```python
from build123d import *

# Parameters (mm, degrees)
F0_W     = 46
F0_H     = 18
F0_W_2   = 40
F0_H_2   = 12
F1_DEPTH = 11
F2_W     = 40
F2_H     = 12
F3_DEPTH = 3
F4_R     = 1


with BuildPart() as f1:
    # F0 (on Top) → F1 (new body)
    with BuildSketch(Plane.XY):
        with Locations((23, 9)):
            Rectangle(F0_W, F0_H)
        with Locations((23, 9)):
            Rectangle(F0_W_2, F0_H_2, mode=Mode.SUBTRACT)
    extrude(amount=F1_DEPTH)

    # F2 (on Top) → F3 (join)
    with BuildSketch(Plane.XY):
        with Locations((23, 9)):
            Rectangle(F2_W, F2_H)
    extrude(amount=F3_DEPTH)

    # F4
    f4_edges = [f1.edges().sort_by_distance(p)[0] for p in [
        (46, 18, 5.5),
        (46, 0, 5.5),
        (0, 0, 5.5),
        (0, 18, 5.5),
        (23, 18, 11),
        (0, 9, 11),
        (23, 0, 11),
        (46, 9, 11),
    ]]
    fillet(f4_edges, radius=F4_R)


solid = f1.part
```
Source: CAD feature listing. Evaluate the final solid. Frame: model axes, mm. A direction names the side the tool comes from. Coordinates: 2 decimals unless noted, no trailing zeros. Loops run counter-clockwise (first coordinate to the right, second up) from the corner with the lowest first, then second, coordinate; pieces in that order, holes last. Notation, with made-up numbers: (21.5, 68) -> (64.5, 68) arc R23 cw to (64.5, 83) -> close; hole circle Ø5 at (-15, 58). An arc over 180 degrees is marked (long way). One line per item, written item: value. Start each with the question number.
Q1. Section query B-B, the plane x = 42.5. Return the cut outline in (y, z), and give its area (3 significant figures).
Q2. Set-up query: faces 4 (the face through (23, 18, 5)), 5 (the face through (23, 9, 3)). Return all of +Z, -Z, +X, -X, +Y, -Y with unobstructed straight access to the full face (end or side cutting, diameter ignored); none if empty.
Q3. Line query: line 1 along Y through (x, z) = (24, 10); line 2 along X through (y, z) = (4.5, 4.5); line 3 along Z through (x, y) = (24.5, 13.5). Output: solid intervals per line, ascending.
Q4. Section query C-C, the plane y = 5.25. Return the cut outline in (x, z).
Q5. Contact query for flat-ended pins moving along their axis: P1, Ø1.5, axis at x = 32, y = 5, coming from the +Z side; P2, Ø6, axis at x = 15.5, y = 14.5, coming from the -Z side. Output: stop coordinate, or through.
Q6. Mould query, pull axis X, two halves, no side actions, for faces 1 (the face through (23, 3, 7)), 2 (the face through (0.285, 17.699, 5.07)), 3 (the face through (23.308, 0.285, 10.699)). Classes: pulls with the +X half, pulls with the -X half, needs draft (parallel to the pull), parting line crosses it, or undercut.
Q7. Section query A-A, the plane z = 9. Return the cut outline in (x, y), and give its area (3 significant figures).
Results:
1. outline: (0, 0) -> (18, 0) -> (18, 10) arc R1 ccw to (17, 11) -> (15, 11) -> (15, 3) -> (3, 3) -> (3, 11) -> (1, 11) arc R1 ccw to (0, 10) -> close
1. area: 102 mm^2
2. face 4: +Z, -Z, +X, -X, +Y
2. face 5: +Z
3. line 1: 0 to 3, 15 to 18
3. line 2: 0 to 3, 43 to 46
3. line 3: 0 to 3
4. outline: (0, 0) -> (46, 0) -> (46, 10) arc R1 ccw to (45, 11) -> (43, 11) -> (43, 3) -> (3, 3) -> (3, 11) -> (1, 11) arc R1 ccw to (0, 10) -> close
5. P1: z = 3
5. P2: z = 0
6. face 1: undercut
6. face 2: pulls with the -X half
6. face 3: needs draft
7. outline: (0, 1) arc R1 ccw to (1, 0) -> (45, 0) arc R1 ccw to (46, 1) -> (46, 17) arc R1 ccw to (45, 18) -> (1, 18) arc R1 ccw to (0, 17) -> close; hole (3, 3) -> (43, 3) -> (43, 15) -> (3, 15) -> close
7. area: 347 mm^2
